Check sheet for the modelled part. Datum: model origin and axes. Units: mm. A direction names the side the tool comes from. Give positions to 0.01 mm unless a question says otherwise; leave off trailing zeros. Order: outer loops, then holes, each group sorted by start corner. A loop starts at its lowest first (then second) coordinate and runs counter-clockwise, first axis right, second up.
from build123d import *

# Parameters (mm, degrees)
CUT_EXTRUDE1_DEPTH      = 62.112017288
CUT_EXTRUDE1_DEPTH_BACK = 62.112017288
SKETCH2_R               = 5
SKETCH3_W               = 1
SKETCH3_H               = 1.5
SKETCH4_W               = 103.716801646
SKETCH4_H               = 65.276308729
CUT_EXTRUDE2_DEPTH      = 40


with BuildPart() as part:
    # Sketch1 one side → Revolve2 (revolve)
    with BuildSketch(Plane.XY, mode=Mode.PRIVATE) as revolve2_sk:
        with BuildLine():
            Line((-30, 42), (-30, 0))
            Line((-30, 0), (-15, 0))
            Line((-15, 0), (-15, 35))
            Line((-15, 35), (-26, 35))
            Line((-26, 35), (-26, 38))
            ThreePointArc((-26, 38), (-13.033669609, 39.403753083), (0, 39.872478009))
            Line((0, 39.872478009), (0, 43.984982176))
            ThreePointArc((0, 43.984982176), (-15.03279876, 43.488194683), (-30, 42))
        make_face()
    revolve(revolve2_sk.sketch.rotate(Axis((0, 45, 0), (0, 1, 0)), 270), axis=Axis((0, 45, 0), (0, 1, 0)))

    # Sketch2 → Cut-Extrude1 (cut, two sides: drawn at the far end of the back side and taken through both)
    with BuildSketch(Plane(origin=(0, 0, 0), x_dir=(0, 0, -1), z_dir=(1, 0, 0)).offset(-CUT_EXTRUDE1_DEPTH_BACK)):
        with Locations((0, 12)):
            Circle(SKETCH2_R)
    extrude(amount=CUT_EXTRUDE1_DEPTH + CUT_EXTRUDE1_DEPTH_BACK, mode=Mode.SUBTRACT)

    # Sketch3 → Cut-Revolve1 (revolve, cut)
    with BuildSketch(Plane(origin=(0, 0, 0), x_dir=(0, 0, -1), z_dir=(1, 0, 0)), mode=Mode.PRIVATE) as cut_revolve1_sk:
        with Locations((29.5, 25.75)):
            Rectangle(SKETCH3_W, SKETCH3_H)
        with Locations((29.5, 30.75)):
            Rectangle(SKETCH3_W, SKETCH3_H)
        with Locations((29.5, 35.75)):
            Rectangle(SKETCH3_W, SKETCH3_H)
    revolve(cut_revolve1_sk.sketch.rotate(Axis((0, 42, 0), (0, -1, 0)), 180), axis=Axis((0, 42, 0), (0, -1, 0)), mode=Mode.SUBTRACT)

    # Sketch4 → Cut-Extrude2 (cut)
    with BuildSketch(Plane.XY):
        with Locations((-0.592885071, 21.596736742)):
            Rectangle(SKETCH4_W, SKETCH4_H)
    extrude(amount=CUT_EXTRUDE2_DEPTH, mode=Mode.SUBTRACT)


solid = part.part
1) Section check C-C, the plane y = 4. Record the cut outline in (x, z).
Recorded:
outline: (-30, 0) arc R30 ccw to (30, 0) - (15, 0) arc R15 cw to (-15, 0) - close
2) Depth check by flat-ended pin: pin 1 Ø13 at (x, z) = (-2, -10.5) entering from +Y; pin 2 Ø3 at (x, z) = (-5, -21) entering from +Y; pin 3 Ø4 at (x, z) = (-15.5, -10.5) entering from +Y. Enter the tip coordinate at first touch or a pass-through.
Recorded:
pin 1: stops at y = 43.95
pin 2: stops at y = 43.1
pin 3: stops at y = 43.37
3) Section check A-A, the plane x = 0. Record the cut outline in (y, z), then the cut area to 3 significant figures.
Recorded:
outline: (0, -30) - (25, -30) - (25, -29) - (26.5, -29) - (26.5, -30) - (30, -30) - (30, -29) - (31.5, -29) - (31.5, -30) - (35, -30) - (35, -29) - (36.5, -29) - (36.5, -30) - (42, -30) arc R227.69 ccw to (43.98, 0) - (39.87, 0) arc R181.45 cw to (38, -26) - (35, -26) - (35, -15) - (0, -15) - close
area: 660 mm2
4) Set-up check for faces 4 (the face through (0, 35, -16)), 5 (the face through (-22, 12, -5)), 6 (the face through (0, 18, -15)), 7 (the face through (-2.4, 35, -29.4)): record each of +Z, -Z, +X, -X, +Y, -Y from which the full face is reachable in a straight line by a thin tool's end or side.
Recorded:
face 4: +Z
face 5: +Z, +X, -X
face 6: +Z, -Y
face 7: -Z
5) Section check D-D, the plane x = 8. Record the cut outline in (y, z).
Recorded:
outline: (0, -28.91) - (25, -28.91) - (25, -27.87) - (26.5, -27.87) - (26.5, -28.91) - (30, -28.91) - (30, -27.87) - (31.5, -27.87) - (31.5, -28.91) - (35, -28.91) - (35, -27.87) - (36.5, -27.87) - (36.5, -28.91) - (42, -28.91) arc R227.55 ccw to (43.84, 0) - (39.7, 0) arc R181.27 cw to (38, -24.74) - (35, -24.74) - (35, -12.69) - (0, -12.69) - close
6) Draft check along Y on faces 1 (the face through (-2.4, 31.5, -29.4)), 2 (the face through (0.66, 39.212, -29.993)), 3 (the face through (0, 0, -18)). Enter one of: +Y half, -Y half, draft (parallel to the pull), parting line (faces both ways), or undercut.
Recorded:
face 1: undercut
face 2: draft
face 3: -Y half
7) Material ranges on L1, parallel to Y at x = 24, z = -16.5; L2, parallel to X at y = 19, z = -9.5; L3, parallel to X at y = 20, z = -6, recorded low to high.
Recorded:
L1: y = 0 to 25, 26.5 to 30, 31.5 to 35, 36.5 to 42.11
L2: x = -28.46 to -11.61, 11.61 to 28.46
L3: x = -29.39 to -13.75, 13.75 to 29.39
